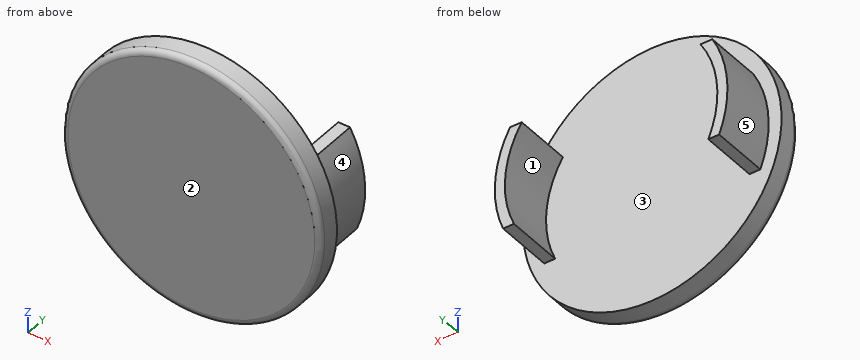
from build123d import *

# Parameters (mm, degrees)
SKETCH1_R           = 22.5
SKETCH1_R_2         = 20.25
SKETCH1_R_3         = 18.5
BOSS_EXTRUDE1_DEPTH = 4
SKETCH2_R           = 20.25
SKETCH2_R_2         = 18.5
BOSS_EXTRUDE2_DEPTH = 10
SKETCH3_W           = 46.515228405
SKETCH3_H           = 15.633520553
SKETCH3_W_2         = 41.010467647
SKETCH3_H_2         = 11.670092807
CUT_EXTRUDE1_DEPTH  = 10
FILLET1_R           = 1


with BuildPart() as part:
    # Sketch1 → Boss-Extrude1 (new body)
    # profile 1 of 3: a face of its own
    with BuildSketch(Plane(origin=(0, 0, 0), x_dir=(1, 0, 0), z_dir=(0, 1, 0))):
        with Locations(Location((0, 0, 0), (0, 0, 270))):
            Circle(SKETCH1_R)
        Circle(SKETCH1_R_2, mode=Mode.SUBTRACT)
    # profile 2 of 3: a face of its own
    with BuildSketch(Plane(origin=(0, 0, 0), x_dir=(1, 0, 0), z_dir=(0, 1, 0))):
        Circle(SKETCH1_R_2)
        Circle(SKETCH1_R_3, mode=Mode.SUBTRACT)
    # profile 3 of 3: a face of its own
    with BuildSketch(Plane(origin=(0, 0, 0), x_dir=(1, 0, 0), z_dir=(0, 1, 0))):
        Circle(SKETCH1_R_3)
    extrude(amount=BOSS_EXTRUDE1_DEPTH)

    # Sketch2 → Boss-Extrude2 (add)
    with BuildSketch(Plane(origin=(0, 4, 0), x_dir=(1, 0, 0), z_dir=(0, 1, 0))):
        with Locations(Location((0, 0, 0), (0, 0, 270))):
            Circle(SKETCH2_R)
        with Locations(Location((0, 0, 0), (0, 0, 270))):
            Circle(SKETCH2_R_2, mode=Mode.SUBTRACT)
    extrude(amount=BOSS_EXTRUDE2_DEPTH)

    # Sketch3 → Cut-Extrude1 (cut)
    with BuildSketch(Plane(origin=(0, 14, 0), x_dir=(1, 0, 0), z_dir=(0, 1, 0))):
        with Locations((-0.927501078, 15.316760277)):
            Rectangle(SKETCH3_W, SKETCH3_H)
        with Locations((-0.707310647, -15.835046403)):
            Rectangle(SKETCH3_W_2, SKETCH3_H_2)
    extrude(amount=-CUT_EXTRUDE1_DEPTH, mode=Mode.SUBTRACT)

    # Fillet1
    fillet1_edges = [part.edges().sort_by_distance(p)[0] for p in [
        (0, 0, -22.5),
    ]]
    fillet(fillet1_edges, radius=FILLET1_R)


solid = part.part
The model under review builds one solid part; all positions refer to its coordinate system, in mm. Face numbers are marked on the shaded views. A direction names the side the tool comes from. Round coordinates to 2 decimals unless told otherwise and drop trailing zeros. Loops run counter-clockwise (first coordinate to the right, second up) from the corner with the lowest first, then second, coordinate; pieces in that order, holes last. Notation, with made-up numbers: (-12.5, -38.5) -> (21.5, -38.5) arc R33 cw to (21.5, -6.5) -> close; hole circle Ø3 at (41, 49). An arc over 180 degrees is marked (long way). One line per question, with ' | ' between items. Start each with the question number.
Item 1: Draft analysis for pull direction X (two halves, no side actions). For the marked faces 3, 4 and 5, state which applies: +X half, -X half, draft (parallel to the pull), parting line (faces both ways), or undercut.
Item 2: Add section A-A, the plane y = 7.75. Write out the cut boundary in (x, z), then the cut area to 3 significant figures.
Item 3: Machinability: for the marked faces 1 and 2, which of the approach directions +Z, -Z, +X, -X, +Y, -Y give a long, thin tool a straight path to every point of the face, cutting with its end or side? Answer none if there is none.
Item 4: For pin 1 (2 mm diameter, centred on x = 16.5, y = 11, fed in from +Z); pin 2 (8 mm diameter, centred on x = 3, z = 3, fed in from +Y); pin 3 (5 mm diameter, centred on x = -1, z = 0.5, fed in from -Y); pin 4 (8 mm diameter, centred on y = 9.5, z = 4, fed in from +X), all flat-tipped, find the tip position at first contact; note any pin that passes through.
Item 5: Wall thickness on line 1 along X through (y, z) = (13, -0.5); line 2 along X through (y, z) = (5, -5); line 3 along Y through (x, z) = (6, 5.5): over which ranges is each line inside the solid? List them lowest first. Write a range as [from, to].
Item 6: Add section B-B, the plane z = 0. Write out the cut boundary in (x, y).
Return value:
1) face 3: undercut | face 4: +X half | face 5: -X half
2) outline: (-18.81, -7.5) -> (-16.91, -7.5) arc R18.5 cw to (-15.56, 10) -> (-17.61, 10) arc R20.25 ccw to start; (15.56, 10) arc R18.5 cw to (16.91, -7.5) -> (18.81, -7.5) arc R20.25 ccw to (17.61, 10) -> close | area: 63.7 mm2
3) face 1: +Y | face 2: +Z, -Z, +X, -X, -Y
4) pin 1: stops at z = 10 | pin 2: stops at y = 4 | pin 3: stops at y = 0 | pin 4: stops at x = 20.25
5) line 1: x = [-20.24, -18.49], [18.49, 20.24] | line 2: x = [-19.62, -17.81], [17.81, 19.62] | line 3: y = [0, 4]
6) outline: (-22.5, 1) arc R1 ccw to (-21.5, 0) -> (21.5, 0) arc R1 ccw to (22.5, 1) -> (22.5, 4) -> (20.25, 4) -> (20.25, 14) -> (18.5, 14) -> (18.5, 4) -> (-18.5, 4) -> (-18.5, 14) -> (-20.25, 14) -> (-20.25, 4) -> (-22.5, 4) -> close
